Check sheet for the modelled part. Datum: model origin and axes. Units: mm. A direction names the side the tool comes from. Give positions to 0.01 mm unless a question says otherwise; leave off trailing zeros. Order: outer loops, then holes, each group sorted by start corner. A loop starts at its lowest first (then second) coordinate and runs counter-clockwise, first axis right, second up. Notation, with made-up numbers: (37, 48) -> (81, 48) arc R19 ccw to (81, 85) -> close; hole circle Ø9 at (-11, -24.5). An arc over 180 degrees is marked (long way). Write each question's results on one line, items separated by ' | '.
from build123d import *

# Parameters (mm, degrees)
SKETCH1_R           = 3
BOSS_EXTRUDE1_DEPTH = 6
BOSS_EXTRUDE2_DEPTH = 3
SKETCH3_R           = 6.85
CUT_EXTRUDE1_DEPTH  = 5.2
SKETCH4_R           = 7.85
CUT_EXTRUDE2_DEPTH  = 1
SKETCH5_R           = 6.85
CUT_EXTRUDE3_DEPTH  = 5.2
SKETCH6_R           = 7.85
CUT_EXTRUDE4_DEPTH  = 1


with BuildPart() as part:
    # Sketch1 → Boss-Extrude1 (new body)
    with BuildSketch(Plane.XY):
        Polygon((12.071067812, 5), (5, 12.071067812), (-5, 12.071067812), (-12.071067812, 5), (-14.676359397, 2.394708415), (-105.323640603, 2.394708415), (-107.928932188, 5), (-115, 12.071067812), (-125, 12.071067812), (-132.071067812, 5), (-132.071067812, -5), (-125, -12.071067812), (-115, -12.071067812), (-107.928932188, -5), (-105.323640603, -2.394708415), (-14.676359397, -2.394708415), (-12.071067812, -5), (-5, -12.071067812), (5, -12.071067812), (12.071067812, -5), align=None)
        with Locations((-120, 0)):
            Circle(SKETCH1_R, mode=Mode.SUBTRACT)
        Circle(SKETCH1_R, mode=Mode.SUBTRACT)
    extrude(amount=-BOSS_EXTRUDE1_DEPTH)

    # Sketch2 → Boss-Extrude2 (add)
    with BuildSketch(Plane.XY):
        Polygon((-14.676359397, -2.394708415), (-12.071067812, -5), (-107.928932188, -5), (-105.323640603, -2.394708415), align=None)
        Polygon((-14.676359397, 2.394708415), (-105.323640603, 2.394708415), (-107.928932188, 5), (-12.071067812, 5), align=None)
    extrude(amount=-BOSS_EXTRUDE2_DEPTH)

    # Sketch3 → Cut-Extrude1 (cut)
    with BuildSketch(Plane(origin=(0, 0, -6), x_dir=(-1, 0, 0), z_dir=(0, 0, -1))):
        Circle(SKETCH3_R)
    extrude(amount=-CUT_EXTRUDE1_DEPTH, mode=Mode.SUBTRACT)

    # Sketch4 → Cut-Extrude2 (cut)
    with BuildSketch(Plane(origin=(0, 0, -6), x_dir=(-1, 0, 0), z_dir=(0, 0, -1))):
        Circle(SKETCH4_R)
    extrude(amount=-CUT_EXTRUDE2_DEPTH, mode=Mode.SUBTRACT)

    # Sketch5 → Cut-Extrude3 (cut)
    with BuildSketch(Plane.XY):
        with Locations((-120, 0)):
            Circle(SKETCH5_R)
    extrude(amount=-CUT_EXTRUDE3_DEPTH, mode=Mode.SUBTRACT)

    # Sketch6 → Cut-Extrude4 (cut)
    with BuildSketch(Plane.XY):
        with Locations((-120, 0)):
            Circle(SKETCH6_R)
    extrude(amount=-CUT_EXTRUDE4_DEPTH, mode=Mode.SUBTRACT)


solid = part.part
1. Mould release check, pull along Y, two halves, no side actions. Record for faces 1 (the flat face through (-59, 2.395, -4)), 2 (the flat face through (-3, -1, -0.8)), 3 (the flat face through (-61, -2.395, -4)): +Y half, -Y half, draft (parallel to the pull), parting line (faces both ways), or undercut.
Verdict:
face 1: +Y half | face 2: undercut | face 3: -Y half
2. Gauge pin test, flat ends, axial feed: pin 1 Ø14 at (x, y) = (0, 0) entering from -Z; pin 2 Ø2.5 at (x, z) = (-79.5, -1) entering from +Y; pin 3 Ø2.5 at (x, z) = (-76.5, -4.5) entering from +Y; pin 4 Ø12 at (x, y) = (-46, 2.5) entering from +Z. Record the tip position at first contact, or that the pin passes through.
Verdict:
pin 1: stops at z = -5 | pin 2: stops at y = 5 | pin 3: stops at y = 2.39 | pin 4: stops at z = 0
3. Section check B-B on x = -120. Record the cut outline in (y, z).
Verdict:
outline: (-12.07, -6) -> (-3, -6) -> (-3, -5.2) -> (-6.85, -5.2) -> (-6.85, -1) -> (-7.85, -1) -> (-7.85, 0) -> (-12.07, 0) -> close; (3, -6) -> (12.07, -6) -> (12.07, 0) -> (7.85, 0) -> (7.85, -1) -> (6.85, -1) -> (6.85, -5.2) -> (3, -5.2) -> close
4. Material ranges on probe 1 along Y at (x, z) = (0, -0.5); probe 2 along Y at (x, z) = (0, -5.75); probe 3 along X at (y, z) = (5.5, -2.55), recorded low to high. Write a range as from..to.
Verdict:
probe 1: y = -12.07..-3, 3..12.07 | probe 2: y = -12.07..-7.85, 7.85..12.07 | probe 3: x = -131.57..-124.08, -115.92..-108.43, -11.57..-4.08, 4.08..11.57
5. Access from +Z, -Z, +X, -X, +Y, -Y to the whole of each face (thin tool, end or side, straight path). Record for faces 4 (the flat face through (-59, -4, -3)), 5 (the cylindrical face through (5.786, 5.305, -5.507)), 6 (the cylindrical face through (-126.843, 0.301, -3.071)).
Verdict:
face 4: -Z, -Y | face 5: -Z | face 6: +Z
6. Section check C-C on y = 0. Record the cut outline in (x, z), then the cut area to 3 significant figures.
Verdict:
outline: (-132.07, -6) -> (-123, -6) -> (-123, -5.2) -> (-126.85, -5.2) -> (-126.85, -1) -> (-127.85, -1) -> (-127.85, 0) -> (-132.07, 0) -> close; (-117, -6) -> (-7.85, -6) -> (-7.85, -5) -> (-6.85, -5) -> (-6.85, -0.8) -> (-3, -0.8) -> (-3, 0) -> (-112.15, 0) -> (-112.15, -1) -> (-113.15, -1) -> (-113.15, -5.2) -> (-117, -5.2) -> close; (3, -0.8) -> (6.85, -0.8) -> (6.85, -5) -> (7.85, -5) -> (7.85, -6) -> (12.07, -6) -> (12.07, 0) -> (3, 0) -> close | area: 709 mm^2
7. Section check A-A on z = -2. Record the cut outline in (x, y).
Verdict:
outline: (-132.07, -5) -> (-125, -12.07) -> (-115, -12.07) -> (-107.93, -5) -> (-12.07, -5) -> (-5, -12.07) -> (5, -12.07) -> (12.07, -5) -> (12.07, 5) -> (5, 12.07) -> (-5, 12.07) -> (-12.07, 5) -> (-107.93, 5) -> (-115, 12.07) -> (-125, 12.07) -> (-132.07, 5) -> close; hole circle Ø13.7 at (-120, 0); hole circle Ø13.7 at (0, 0)
8. Section check D-D on y = 9.75. Record the cut outline in (x, z), then the cut area to 3 significant figures.
Verdict:
outline: (-127.32, -6) -> (-112.68, -6) -> (-112.68, 0) -> (-127.32, 0) -> close; (-7.32, -6) -> (7.32, -6) -> (7.32, 0) -> (-7.32, 0) -> close | area: 176 mm^2
